```python
from build123d import *

# Parameters (mm, degrees)
F0_W          = 279.4
F0_H          = 482.6
F1_DEPTH      = 190.5
F2_T          = -2.54
F3_W          = 13.208
F3_H          = 12.7
F4_DEPTH      = 0.0254
F4_DEPTH_BACK = 33.02


with BuildPart() as f1:
    # F0 (on Front) → F1 (new body, symmetric)
    with BuildSketch(Plane.XZ):
        Rectangle(F0_W, F0_H)
    extrude(amount=F1_DEPTH, both=True)

    # F2
    f2_openings = [f1.faces().sort_by_distance(p)[0] for p in [
        (0, -190.5, 0),
    ]]
    offset(amount=F2_T, openings=f2_openings)

    # F3 (on face) → F4 (join, two sides)
    with BuildSketch(Plane.YZ.offset(139.7)) as f4_sk:
        with Locations((-165.152445, 30.9372)):
            Rectangle(F3_W, F3_H)
    extrude(amount=F4_DEPTH)
    extrude(f4_sk.sketch, amount=-F4_DEPTH_BACK)


solid = f1.part
```
The model under review builds one solid part; all positions refer to its coordinate system, in mm. A direction names the side the tool comes from. Give positions to 0.01 mm unless a question says otherwise; leave off trailing zeros. Write each loop counter-clockwise with the first axis right and the second up, starting at its lowest first coordinate (ties: lowest second). Pieces come first, ordered by that corner, then holes. Notation, with made-up numbers: M 9,-26.75 L 43,-26.75 A21 ccw 43,-6.75 Z; hole C 67.5,-29.75 d2. An arc over 180 degrees is marked long. Write each question's results on one line, items separated by ' | '. Start each with the question number.
1. For probe 1 along X at (y, z) = (113, 73.5); probe 2 along Z at (x, y) = (16, 147); probe 3 along Y at (x, z) = (-117.5, -102), list the stretches that pass through material, from the lowest coordinate up. Write a range as [from, to].
2. Mouldability with a two-part tool opening along Z and no side actions: class faces 4 (the flat face through (139.725, -165, 31)), 5 (the flat face through (-2, -3, -241.3)), 6 (the flat face through (122, -171.756, 31)) as released by +Z, released by -Z, zero draft, split by the parting line, or undercut.
3. Insertion check: pin 1 Ø3 at (y, z) = (74.5, 73.5) entering from +X; pin 2 Ø6 at (x, z) = (72, 4) entering from -Y; pin 3 Ø14 at (x, z) = (128.5, 33) entering from -Y. Each pin has a flat end and moves straight along its axis. Give the tip position at first contact, or say it passes through.
4. For faces 1 (the flat face through (122, -158.548, 31)), 2 (the flat face through (-2, -4, 238.76)), 3 (the flat face through (139.7, -3, -3)), list the 3-axis set-ups (+Z, -Z, +X, -X, +Y, -Y) from which the entire face can be reached by the end or side of a thin tool; tool diameter is ignored.
5. We need section A-A (y = 168). Write out the cut boundary in (x, z), and give its area (3 significant figures).
6. We need section B-B (z = 124). Write out the cut boundary in (x, y).
7. We need section C-C (x = -120). Write out the cut boundary in (y, z).
Results found:
1) probe 1: x = [-139.7, -137.16], [137.16, 139.7] | probe 2: z = [-241.3, -238.76], [238.76, 241.3] | probe 3: y = [187.96, 190.5]
2) face 4: zero draft | face 5: released by -Z | face 6: undercut
3) pin 1: stops at x = 139.7 | pin 2: stops at y = 187.96 | pin 3: stops at y = -171.76
4) face 1: none | face 2: -Y | face 3: +Z, -Z, +X, +Y, -Y
5) outline: M -139.7,-241.3 L 139.7,-241.3 L 139.7,241.3 L -139.7,241.3 Z; hole M -137.16,-238.76 L 137.16,-238.76 L 137.16,238.76 L -137.16,238.76 Z | area: 3,850 mm^2
6) outline: M -139.7,-190.5 L -137.16,-190.5 L -137.16,187.96 L 137.16,187.96 L 137.16,-190.5 L 139.7,-190.5 L 139.7,190.5 L -139.7,190.5 Z
7) outline: M -190.5,-241.3 L 190.5,-241.3 L 190.5,241.3 L -190.5,241.3 L -190.5,238.76 L 187.96,238.76 L 187.96,-238.76 L -190.5,-238.76 Z
